```python
from build123d import *

# Parameters (mm, degrees)
EXTRUDE_1_DEPTH     = 4
CUT_EXTRUDE_1_DEPTH = 1.5
CUT_EXTRUDE_2_DEPTH = 6


with BuildPart() as part:
    # Эскиз1 → Бобышка-Вытянуть1 (new body, symmetric)
    with BuildSketch(Plane.XY):
        Polygon((4, 0), (-4, 0), (-4, -1.5), (-8, -1.5), (-8, -6.5), (8, -6.5), (8, -1.5), (4, -1.5), align=None)
    extrude(amount=EXTRUDE_1_DEPTH, both=True)

    # Эскиз3 → Отверстие обработанное метчиком M61 (revolve, cut)
    with BuildSketch(Plane(origin=(0, 0, 0), x_dir=(0, 0, 1), z_dir=(1, 0, 0))):
        Polygon((0, 0), (0, 6.5), (3.5, 6.5), (2.5, 5.5), (2.5, 1), (3.5, 0), align=None)
    revolve(axis=Axis((0, 6.35, 0), (0, -1, 0)), mode=Mode.SUBTRACT)

    # Эскиз4 → Вырез-Вытянуть1 (cut)
    with BuildSketch(Plane(origin=(0, 0, 0), x_dir=(1, 0, 0), z_dir=(0, 1, 0))):
        with BuildLine():
            Line((-4, 4), (-4, 0))
            ThreePointArc((-4, 0), (-2.828427125, 2.828427125), (0, 4))
            Line((0, 4), (-4, 4))
        make_face()
        with BuildLine():
            Line((0, -4), (4, -4))
            Line((4, -4), (4, 0))
            ThreePointArc((4, 0), (2.828427125, -2.828427125), (0, -4))
        make_face()
    extrude(amount=-CUT_EXTRUDE_1_DEPTH, mode=Mode.SUBTRACT)

    # Эскиз5 → Вырез-Вытянуть2 (cut, through all)
    with BuildSketch(Plane(origin=(0, -1.5, 0), x_dir=(1, 0, 0), z_dir=(0, 1, 0))):
        with BuildLine():
            Line((-8, 0), (-8, 4))
            Line((-8, 4), (-6.92820323, 4))
            ThreePointArc((-6.92820323, 4), (-7.72740661, 2.070552361), (-8, 0))
        make_face()
        with BuildLine():
            Line((8, 0), (8, -4))
            Line((8, -4), (6.92820323, -4))
            ThreePointArc((6.92820323, -4), (7.72740661, -2.070552361), (8, 0))
        make_face()
    extrude(amount=-CUT_EXTRUDE_2_DEPTH, mode=Mode.SUBTRACT)

    # Вырез-По траектории1: sweep along a path in Эскиз7
    with BuildLine(Plane.XZ.offset(6.5)) as sweep_1_path:
        Line((0, 8), (-8, 8))
        Line((-8, 8), (-8, 0))
        ThreePointArc((-8, 0), (-5.656854249, -5.656854249), (0, -8))
        Line((0, -8), (8, -8))
        Line((8, -8), (8, 0))
        ThreePointArc((8, 0), (5.656854249, 5.656854249), (0, 8))
    # Эскиз6 → Вырез-По траектории1 (sweep, cut)
    with BuildSketch(Plane.XY.offset(4)):
        Polygon((-8, -3), (-8, -6.5), (-4, -6.5), align=None)
    sweep(path=sweep_1_path.line, transition=Transition.RIGHT, mode=Mode.SUBTRACT)


solid = part.part
```
Input: part model. Units: mm. Frame: model coordinates. A direction names the side the tool comes from. Give positions to 0.01 mm unless a question says otherwise; leave off trailing zeros. Write item = value, one per line. Start each with the question number.
1) Draft query along X for faces 4 (the face through (2.859, -0.74, 2.797)), 5 (the face through (-2.859, -0.74, -2.797)), 6 (the face through (-3, -6, 0)), 7 (the face through (-1, -3, 4)). Return one class per face: pulls with the +X half, pulls with the -X half, needs draft (parallel to the pull), parting line crosses it, or undercut.
2) Reachability of faces 1 (the face through (-4, -1, 2)), 2 (the face through (-6, -1.5, 0)), 3 (the face through (5.972, -4.774, -1.972)) from +Z, -Z, +X, -X, +Y, -Y: full face, straight path, thin tool, end or side. Return the list, or none.
3) Pin query (flat end, axial travel): pin 1 (2.5 mm diameter, centred on x = -5, z = -2, fed in from +Y). Return the tip coordinate at first contact, or that it passes through.
4) Material intervals for L1, parallel to Z at x = 0, y = -2.95; L2, parallel to X at y = -2.25, z = 0; L3, parallel to Z at x = -1, y = -3.75, sorted ascending. Write a range as [from, to].
Answers follow:
q1.face_4 = pulls with the +X half
q1.face_5 = pulls with the -X half
q1.face_6 = undercut
q1.face_7 = needs draft
q2.face_1 = +Z, -Z, -X, +Y
q2.face_2 = -Z, -X, +Y
q2.face_3 = +Z, -Z, +X, -Y
q3.pin_1 = -1.5
q4.L1 = [-4, -2.5], [2.5, 4]
q4.L2 = [-8, -2.5], [2.5, 8]
q4.L3 = [-4, -2.29], [2.29, 4]
